Geometry check sheet. Reference: the model listing, model coordinates, mm. Face numbers are marked on the shaded views. Coordinates: 2 decimals unless noted, no trailing zeros. Order: outer loops, then holes, each group sorted by start corner. A loop starts at its lowest first (then second) coordinate and runs counter-clockwise, first axis right, second up. Notation, with made-up numbers: (60.5, -7) - (90.5, -7) arc R24 cw to (90.5, 23) - close; hole circle Ø4 at (5, 26.5). An arc over 180 degrees is marked (long way). Put each result on its own line as item: value.
from build123d import *

# Parameters (mm, degrees)
SKETCH1_W              = 75
SKETCH1_H              = 75
BOSS_EXTRUDE1_DEPTH    = 4.7625
M8_CLEARANCE_HOLE1_D   = 9
M12X1_5_TAPPED_HOLE1_D = 10.5
CHAMFER1_SIZE          = 1


with BuildPart() as part:
    # Sketch1 → Boss-Extrude1 (new, symmetric)
    with BuildSketch(Plane(origin=(0, 0, 0), x_dir=(1, 0, 0), z_dir=(0, 1, 0))):
        Rectangle(SKETCH1_W, SKETCH1_H)
    extrude(amount=BOSS_EXTRUDE1_DEPTH, both=True)

    # M8 Clearance Hole1 (through all)
    with Locations(Plane(origin=(0, 4.7625, 0), x_dir=(1, 0, 0), z_dir=(0, 1, 0))):
        with Locations((-20, 20), (20, 20), (-20, -20), (20, -20)):
            Hole(M8_CLEARANCE_HOLE1_D / 2)

    # M12x1.5 Tapped Hole1 (through all)
    with Locations(Plane(origin=(0, 4.7625, 0), x_dir=(1, 0, 0), z_dir=(0, 1, 0))):
        with Locations((0, 0)):
            Hole(M12X1_5_TAPPED_HOLE1_D / 2)

    # Chamfer1
    chamfer1_edges = [part.edges().sort_by_distance(p)[0] for p in [
        (37.5, 0, 37.5),
        (-37.5, 0, 37.5),
        (-37.5, 0, -37.5),
        (37.5, 0, -37.5),
    ]]
    chamfer(chamfer1_edges, length=CHAMFER1_SIZE)


solid = part.part
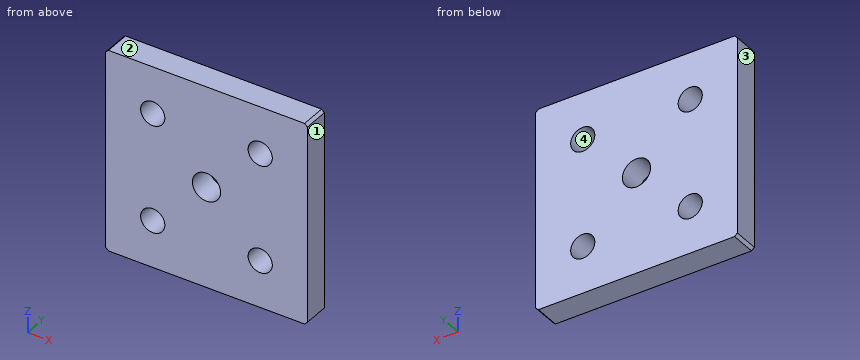
Q1. Thickness scan on L1, parallel to X at y = -2.75, z = 20; L2, parallel to X at y = -4, z = 19. Record the ranges inside material, lowest first. Write a range as [from, to].
Answer block:
L1: x = [-37.5, -24.5], [-15.5, 15.5], [24.5, 37.5]
L2: x = [-37.5, -24.39], [-15.61, 15.61], [24.39, 37.5]
Q2. Section check C-C on y = -3. Record the boundary of the cut face in (x, z).
Answer block:
outline: (-37.5, -36.5) - (-36.5, -37.5) - (36.5, -37.5) - (37.5, -36.5) - (37.5, 36.5) - (36.5, 37.5) - (-36.5, 37.5) - (-37.5, 36.5) - close; hole circle Ø9 at (-20, -20); hole circle Ø9 at (-20, 20); hole circle Ø10.5 at (0, 0); hole circle Ø9 at (20, -20); hole circle Ø9 at (20, 20)
Q3. Draft check along X on the marked faces 1, 2, 3 and 4. Enter one of: pulls with the +X half, pulls with the -X half, needs draft (parallel to the pull), parting line crosses it, or undercut.
Answer block:
face 1: pulls with the +X half
face 2: needs draft
face 3: pulls with the -X half
face 4: undercut
Q4. Section check A-A on x = -20. Record the boundary of the cut face in (y, z), then the cut area to 3 significant figures.
Answer block:
outline: (-4.76, -37.5) - (4.76, -37.5) - (4.76, -24.5) - (-4.76, -24.5) - close; (-4.76, -15.5) - (4.76, -15.5) - (4.76, 15.5) - (-4.76, 15.5) - close; (-4.76, 24.5) - (4.76, 24.5) - (4.76, 37.5) - (-4.76, 37.5) - close
area: 543 mm^2
Q5. Section check D-D on z = 0. Record the boundary of the cut face in (x, y).
Answer block:
outline: (-37.5, -4.76) - (-5.25, -4.76) - (-5.25, 4.76) - (-37.5, 4.76) - close; (5.25, -4.76) - (37.5, -4.76) - (37.5, 4.76) - (5.25, 4.76) - close
Q6. Section check B-B on z = 20. Record the boundary of the cut face in (x, y).
Answer block:
outline: (-37.5, -4.76) - (-24.5, -4.76) - (-24.5, 4.76) - (-37.5, 4.76) - close; (-15.5, -4.76) - (15.5, -4.76) - (15.5, 4.76) - (-15.5, 4.76) - close; (24.5, -4.76) - (37.5, -4.76) - (37.5, 4.76) - (24.5, 4.76) - close
